```python
from build123d import *

# Parameters (mm, degrees)
F1_DEPTH = 20


# Not quite as in the source:
# - a feature names something its author has since deleted; it is built from what else it names


with BuildPart() as f1:
    # F0 (on Front) → F1 (new body)
    with BuildSketch(Plane.XZ):
        with BuildLine():
            ThreePointArc((-18, 68.354232338), (-4.472135955, 96.5656189147), (20, 77.072030225))
            ThreePointArc((20, 77.072030225), (19.4935886896, 72.59989427), (18, 68.354232338))
            Line((18, 68.354232338), (18, 62.7542091618))
            ThreePointArc((18, 62.7542091618), (21.7140507506, 69.489154781), (23, 77.072030225))
            ThreePointArc((23, 77.072030225), (-7.5828754441, 98.7860809757), (-18, 62.7542091618))
            Line((-18, 62.7542091618), (-18, 68.354232338))
        make_face()
        with BuildLine():
            ThreePointArc((-15, 63.8432736697), (-16.6534436987, 65.9967057163), (-18, 68.354232338))
            Line((-18, 68.354232338), (-18, 62.7542091618))
            ThreePointArc((-18, 62.7542091618), (-16.5734766958, 61.1246207109), (-15, 59.6364344509))
            Line((-15, 59.6364344509), (-15, 63.8432736697))
        make_face()
        with BuildLine():
            Line((18, 62.7542091618), (18, 68.354232338))
            ThreePointArc((18, 68.354232338), (16.6534436987, 65.9967057163), (15, 63.8432736697))
            Line((15, 63.8432736697), (15, 59.6364344509))
            ThreePointArc((15, 59.6364344509), (16.5734766958, 61.1246207109), (18, 62.7542091618))
        make_face()
        with BuildLine():
            ThreePointArc((15, 63.8432736697), (0, 57.072030225), (-15, 63.8432736697))
            Line((-15, 63.8432736697), (-15, 59.6364344509))
            ThreePointArc((-15, 59.6364344509), (0, 54.072030225), (15, 59.6364344509))
            Line((15, 59.6364344509), (15, 63.8432736697))
        make_face()
        with BuildLine():
            ThreePointArc((-15, 59.6364344509), (-16.5734766958, 61.1246207109), (-18, 62.7542091618))
            Line((-18, 62.7542091618), (-18, -72.927969775))
            Line((-18, -72.927969775), (18, -72.927969775))
            Line((18, -72.927969775), (18, 62.7542091618))
            ThreePointArc((18, 62.7542091618), (16.5734766958, 61.1246207109), (15, 59.6364344509))
            Line((15, 59.6364344509), (15, -69.927969775))
            Line((15, -69.927969775), (-15, -69.927969775))
            Line((-15, -69.927969775), (-15, 59.6364344509))
        make_face()
    extrude(amount=F1_DEPTH)


solid = f1.part
```
Geometry: final body of the model. Coordinates: model frame, mm. A direction names the side the tool comes from. Round coordinates to 2 decimals unless told otherwise and drop trailing zeros. Write each loop counter-clockwise with the first axis right and the second up, starting at its lowest first coordinate (ties: lowest second). Pieces come first, ordered by that corner, then holes. Notation, with made-up numbers: (52, 38) -> (87, 38) arc R20 cw to (87, 71) -> close; hole circle Ø9 at (-18.75, 66.5). An arc over 180 degrees is marked (long way). Return JSON: item names as keys, results as strings.
Q1. Set-up query: faces 1 (the flat face through (-18, -10, -4)), 2 (the flat face through (18, -10, -6)), 3 (the flat face through (-15.4, 0, 26.8)), 4 (the flat face through (0, -10, -69.928)). Return all of +Z, -Z, +X, -X, +Y, -Y with unobstructed straight access to the full face (end or side cutting, diameter ignored); none if empty.
From the geometry:
{"face 1": "-Z, -X, +Y, -Y", "face 2": "-Z, +X, +Y, -Y", "face 3": "+Z, -Z, +X, -X, +Y", "face 4": "+Y, -Y"}
Q2. Mould query, pull axis Z, two halves, no side actions, for faces 5 (the cylindrical face through (-0.229, -9.86, 54.073)), 6 (the flat face through (0, -10, -72.928)), 7 (the cylindrical face through (0.72, -9.86, 100.06)). Classes: +Z half, -Z half, draft (parallel to the pull), parting line (faces both ways), or undercut.
From the geometry:
{"face 5": "undercut", "face 6": "-Z half", "face 7": "parting line"}
Q3. Section D-D on z = 85.5. Return the cut outline in (x, y).
From the geometry:
{"outline": "(-21.4, -20) -> (-18.14, -20) -> (-18.14, 0) -> (-21.4, 0) -> close; (18.14, -20) -> (21.4, -20) -> (21.4, 0) -> (18.14, 0) -> close"}
Q4. Ray query, line 1 (Z direction, x = -1, y = -8); line 2 (X direction, y = -18.25, z = -2); line 3 (X direction, y = -2.5, z = 77). Return the intervals inside material, ascending.
From the geometry:
{"line 1": "-72.93 to -69.93, 54.09 to 57.1, 97.05 to 100.05", "line 2": "-18 to -15, 15 to 18", "line 3": "-23 to -20, 20 to 23"}
Q5. Section B-B on x = 0. Return the cut outline in (y, z).
From the geometry:
{"outline": "(-20, -72.93) -> (0, -72.93) -> (0, -69.93) -> (-20, -69.93) -> close; (-20, 54.07) -> (0, 54.07) -> (0, 57.07) -> (-20, 57.07) -> close; (-20, 97.07) -> (0, 97.07) -> (0, 100.07) -> (-20, 100.07) -> close"}
Q6. First-contact query: pin 1 Ø10 at (y, z) = (-9, -20.5) entering from +X; pin 2 Ø3 at (x, y) = (6, -9) entering from +Z; pin 3 Ø10 at (y, z) = (-7.5, -16) entering from -X. Flat tips, straight axial feed; report the tip coordinate or a pass-through.
From the geometry:
{"pin 1": "x = 18", "pin 2": "z = 99.63", "pin 3": "x = -18"}
Q7. Section C-C on z = -42. Return the cut outline in (x, y), and give its area (3 significant figures).
From the geometry:
{"outline": "(-18, -20) -> (-15, -20) -> (-15, 0) -> (-18, 0) -> close; (15, -20) -> (18, -20) -> (18, 0) -> (15, 0) -> close", "area": "120 mm2"}
Q8. Section A-A on y = -17.5. Return the cut outline in (x, z), and give its area (3 significant figures).
From the geometry:
{"outline": "(-18, -72.93) -> (18, -72.93) -> (18, 62.75) arc R23 ccw (long way) to (-18, 62.75) -> close; hole circle Ø40 at (0, 77.07); hole (-15, -69.93) -> (15, -69.93) -> (15, 59.64) arc R23 cw to (-15, 59.64) -> close", "area": "1,300 mm2"}
